```python
from build123d import *

# Parameters (mm, degrees)
F1_DEPTH        = 44.45
F3_DEPTH        = 7.874
F5_DEPTH        = 33.274
F7_DEPTH        = 7.874
F9_D            = 12.7
F9_CBORE_D      = 19.05
F9_CBORE_DEPTH  = 20.574
F11_D           = 12.7
F11_START       = 7.874
F11_CBORE_D     = 19.05
F11_CBORE_DEPTH = 20.574
F12_W           = 19.1008
F12_H           = 3.048
F13_DEPTH       = 107.951
F14_SIZE2       = 9.0921120392
F14_SIZE        = 15.748


with BuildPart() as f1:
    # F0 (on Front) → F1 (new body)
    with BuildSketch(Plane.XZ):
        Polygon((0, 69.85), (0, 0), (50.8254, 0), (50.8254, -3.048), (69.85, -3.048), (69.85, 0), (107.95, 0), (107.95, 28.702), (86.0188790381, 28.702), (86.0188790381, 36.576), (44.45, 36.576), (44.45, 69.85), align=None)
    extrude(amount=F1_DEPTH)

    # F2 (on face) → F3 (cut, through all)
    with BuildSketch(Plane.XY.offset(36.576)):
        with BuildLine():
            Line((86.0188790381, 0), (85.8631742014, 0))
            ThreePointArc((85.8631742014, 0), (82.55, -22.225), (85.8631742014, -44.45))
            Line((85.8631742014, -44.45), (86.0188790381, -44.45))
            Line((86.0188790381, -44.45), (86.0188790381, 0))
        make_face()
    extrude(amount=-F3_DEPTH, mode=Mode.SUBTRACT)

    # F4 (on face) → F5 (cut, through all)
    with BuildSketch(Plane.XY.offset(69.85)):
        with BuildLine():
            Line((44.45, -44.45), (44.45, 0))
            ThreePointArc((44.45, 0), (42.2684167521, -22.225), (44.45, -44.45))
        make_face()
    extrude(amount=-F5_DEPTH, mode=Mode.SUBTRACT)

    # F6 (on face) → F7 (cut)
    with BuildSketch(Plane.XY.offset(36.576)):
        with BuildLine():
            Line((44.45, 0), (39.5340062096, 0))
            ThreePointArc((39.5340062096, 0), (37.442416752, -22.225), (39.5340062096, -44.45))
            Line((39.5340062096, -44.45), (44.45, -44.45))
            ThreePointArc((44.45, -44.45), (42.2684167521, -22.225), (44.45, 0))
        make_face()
    extrude(amount=F7_DEPTH, mode=Mode.SUBTRACT)

    # F9 (through all)
    with Locations(Plane.XY.offset(69.85)):
        with Locations((25.4, -22.098)):
            CounterBoreHole(F9_D / 2, F9_CBORE_D / 2, F9_CBORE_DEPTH)

    # F11 (through all)
    # its depths count from where the whole tool has entered the part; down to there all is cleared
    with Locations(Plane.XY.offset(36.576).offset(-F11_START)):
        with Locations((88.9, -22.098)):
            CounterBoreHole(F11_D / 2, F11_CBORE_D / 2, F11_CBORE_DEPTH)

    # F12 (on face) → F13 (cut, through all)
    with BuildSketch(Plane.YZ.offset(107.95)):
        with Locations((-22.1996, 1.524)):
            Rectangle(F12_W, F12_H)
        with Locations((-22.1996, -1.524)):
            Rectangle(F12_W, F12_H)
    extrude(amount=-F13_DEPTH, mode=Mode.SUBTRACT)

    # F14
    f14_edges = [f1.edges().sort_by_distance(p)[0] for p in [
        (0, -22.225, 69.85),
    ]]
    f14_side = f1.faces().sort_by_distance((0, -22.225485, 35.563276))[0]
    chamfer(f14_edges, length=F14_SIZE, length2=F14_SIZE2, reference=f14_side)


solid = f1.part
```
Here's how the part is built. I have some questions about the finished solid (model axes, mm). A direction names the side the tool comes from. Give positions to 0.01 mm unless a question says otherwise; leave off trailing zeros. Loops run counter-clockwise (first coordinate to the right, second up) from the corner with the lowest first, then second, coordinate; pieces in that order, holes last. Notation, with made-up numbers: M -9.75,-0.5 L 20.25,-0.5 A7 ccw 20.25,8.5 Z; hole C -39,-31 d7. An arc over 180 degrees is marked long. Put each result on its own line as item: value. Start each with the question number.
(1) If we mould it in two halves opening along X, with no side actions, what happens to faces 1 (the cylindrical face through (22.47, -27.73, 25.84)), 2 (the flat face through (50.825, -38, -2)), 3 (the flat face through (69.85, -6, -2))? For each: +X half, -X half, draft (parallel to the pull), parting line (faces both ways), or undercut.
(2) I want a section at D-D on x = 88.9. Please give me the cut outline in (y, z), then the cut area to 3 significant figures.
(3) For faces 4 (the flat face through (25, -38, 0)), 5 (the cylindrical face through (15.884, -21.679, 59.707)), 6 (the cylindrical face through (83.985, -36.941, 32.694)), which set-ups out of +Z, -Z, +X, -X, +Y, -Y let a thin tool reach every point of the face, with its end or its side?
(4) Will these pins go through, and if not, where does the flat tip stop? pin 1 Ø13.5 at (x, y) = (53.5, -14.5) entering from +Z; pin 2 Ø3 at (x, y) = (38.5, -30.5) entering from -Z; pin 3 Ø3.5 at (y, z) = (-39, -2) entering from -X.
(5) I want a section at C-C on z = 51. Please give me the cut outline in (x, y) (3 decimals), then the cut area to 3 significant figures.
(6) I want a section at B-B on y = -27. Please give me the cut outline in (x, z).
(7) I need wall thicknesses on line 1 along Y through (x, z) = (25, 57); line 2 along Y through (x, z) = (25, 33); line 3 along Z through (x, y) = (73, -8.5). Which ranges of each line are inside material? Lowest first, please. Write a range as [from, to].
(8) I want a section at A-A on x = 25.4. Please give me the cut outline in (y, z), then the cut area to 3 significant figures.
Answer block:
1. face 1: undercut
1. face 2: -X half
1. face 3: +X half
2. outline: M -44.45,0 L -31.75,0 L -31.75,3.05 L -28.45,3.05 L -28.45,8.13 L -31.62,8.13 L -31.62,28.7 L -44.45,28.7 Z; M -15.75,3.05 L -12.65,3.05 L -12.65,0 L 0,0 L 0,28.7 L -12.57,28.7 L -12.57,8.13 L -15.75,8.13 Z
2. area: 761 mm^2
3. face 4: -Z, -X, +Y, -Y
3. face 5: +Z
3. face 6: +Z, +X
4. pin 1: z = 36.58
4. pin 2: z = 0
4. pin 3: x = 50.83
5. outline: M 0,-44.45 L 44.45,-44.45 A114.3 cw 44.45,0 L 0,0 Z; hole C 25.4,-22.098 d19.05
5. area: 1,630 mm^2
6. outline: M 0,3.05 L 21.36,3.05 L 21.36,49.28 L 17.23,49.28 L 17.23,69.85 L 9.09,69.85 L 0,54.1 Z; M 29.44,3.05 L 84.86,3.05 L 84.86,8.13 L 80.73,8.13 L 80.73,36.58 L 37.54,36.58 L 37.54,44.45 L 42.37,44.45 L 42.37,69.85 L 33.57,69.85 L 33.57,49.28 L 29.44,49.28 Z; M 92.94,3.05 L 107.95,3.05 L 107.95,28.7 L 97.07,28.7 L 97.07,8.13 L 92.94,8.13 Z
7. line 1: [-44.45, -31.61], [-12.58, 0]
7. line 2: [-44.45, -28.44], [-15.76, 0]
7. line 3: [0, 36.58]
8. outline: M -44.45,0 L -31.75,0 L -31.75,3.05 L -28.45,3.05 L -28.45,49.28 L -31.62,49.28 L -31.62,69.85 L -44.45,69.85 Z; M -15.75,3.05 L -12.65,3.05 L -12.65,0 L 0,0 L 0,69.85 L -12.57,69.85 L -12.57,49.28 L -15.75,49.28 Z
8. area: 2,070 mm^2
